CAD build for the part. Positions are in the model's coordinates, mm. A direction names the side the tool comes from. Round coordinates to 2 decimals unless told otherwise and drop trailing zeros. Loops run counter-clockwise (first coordinate to the right, second up) from the corner with the lowest first, then second, coordinate; pieces in that order, holes last.
from build123d import *

# Parameters (mm, degrees)
F0_W     = 40
F0_H     = 40
F0_W_2   = 34.8
F0_H_2   = 34.8
F1_DEPTH = 570
F2_R     = 2
F3_R     = 4


with BuildPart() as f1:
    # F0 (on Front) → F1 (new body)
    with BuildSketch(Plane.XZ):
        Rectangle(F0_W, F0_H)
        Rectangle(F0_W_2, F0_H_2, mode=Mode.SUBTRACT)
    extrude(amount=F1_DEPTH)

    # F2
    f2_edges = [f1.edges().sort_by_distance(p)[0] for p in [
        (-17.4, -285, -17.4),
        (-17.4, -285, 17.4),
        (17.4, -285, 17.4),
        (17.4, -285, -17.4),
    ]]
    fillet(f2_edges, radius=F2_R)

    # F3
    f3_edges = [f1.edges().sort_by_distance(p)[0] for p in [
        (20, -285, 20),
        (-20, -285, 20),
        (20, -285, -20),
        (-20, -285, -20),
    ]]
    fillet(f3_edges, radius=F3_R)


solid = f1.part
Item 1: Cut at A-A (x = 8.5). List the corners of the cut face in (y, z).
Verdict:
outline: (-570, -20) - (0, -20) - (0, -17.4) - (-570, -17.4) - close; (-570, 17.4) - (0, 17.4) - (0, 20) - (-570, 20) - close
Item 2: Cut at C-C (z = 2). List the corners of the cut face in (x, y).
Verdict:
outline: (-20, -570) - (-17.4, -570) - (-17.4, 0) - (-20, 0) - close; (17.4, -570) - (20, -570) - (20, 0) - (17.4, 0) - close
Item 3: Cut at B-B (y = -393). List the corners of the cut face in (x, z), plus the area to 3 significant figures.
Verdict:
outline: (-20, -16) arc R4 ccw to (-16, -20) - (16, -20) arc R4 ccw to (20, -16) - (20, 16) arc R4 ccw to (16, 20) - (-16, 20) arc R4 ccw to (-20, 16) - close; hole (-17.4, -15.4) arc R2 ccw to (-15.4, -17.4) - (15.4, -17.4) arc R2 ccw to (17.4, -15.4) - (17.4, 15.4) arc R2 ccw to (15.4, 17.4) - (-15.4, 17.4) arc R2 ccw to (-17.4, 15.4) - close
area: 379 mm2
Item 4: 3-axis set-ups, long thin cutter, end or side, ignore diameter. For faces 5 (the flat face through (17.4, -281, 0)), 6 (the flat face through (20, -281, 0)): which of +Z, -Z, +X, -X, +Y, -Y reach the whole face in a straight line?
Verdict:
face 5: +Y, -Y
face 6: +Z, -Z, +X, +Y, -Y
Item 5: Wall check: L1, parallel to Z at x = 13, y = -85; L2, parallel to X at y = -172, z = -16. Give the ranges that are in metal, low to high.
Verdict:
L1: z = -20 to -17.4, 17.4 to 20
L2: x = -20 to -17.31, 17.31 to 20
Item 6: Mould opens along Z. For faces 1 (the flat face through (-18, -570, 0)), 2 (the flat face through (0, -281, 17.4)), 3 (the flat face through (0, -281, 20)), 4 (the flat face through (-17.4, -281, 0)) say: released by +Z, released by -Z, zero draft, split by the parting line, or undercut.
Verdict:
face 1: zero draft
face 2: undercut
face 3: released by +Z
face 4: undercut
